Part model, mm, in its own coordinate system. Coordinates: 2 decimals unless noted, no trailing zeros. Order: outer loops, then holes, each group sorted by start corner. A loop starts at its lowest first (then second) coordinate and runs counter-clockwise, first axis right, second up.
1) Pin check, flat tips, straight feed: pin 1 Ø2 at (y, z) = (5.5, 158.5) entering from -X; pin 2 Ø1.5 at (x, y) = (-2.5, 6) entering from +Z; pin 3 Ø4 at (y, z) = (11, 253.5) entering from +X. Stop position of each tip, or through.
2) Wall check: L1, parallel to Y at x = -2.5, z = 331; L2, parallel to Z at x = -2.25, y = 5.5; L3, parallel to X at y = 6.5, z = 51. Give the ranges that are in metal, low to high.
3) Cut at A-A (z = 213). List the corners of the cut face in (x, y).
4) Cut at B-B (z = 30). List the corners of the cut face in (x, y), and give its area (3 significant figures).
Autodesk Inventor part; units mm, degrees
ref_plane "YZ Plane" through (0, 0, 0) normal (1, 0, 0) x (0, 1, 0)
ref_plane "XZ Plane" through (0, 0, 0) normal (0, 1, 0) x (-1, 0, 0)
ref_plane "XY Plane" through (0, 0, 0) normal (0, 0, 1) x (1, 0, 0)
sketch "Sketch1" plane through (0, 0, 0) normal (0, 0, 1) x (1, 0, 0)
  circle A0 centre (-2.6438, 6.9447) radius 6.8758
  line L0 (-9.4616, 7.8359) -> (-6.8245, 12.4034)
  line L1 (-6.8245, 1.4859) -> (-9.4616, 6.0534)
  line L2 (-0.0068, 0.5947) -> (-5.2808, 0.5947)
  line L3 (4.174, 6.0534) -> (1.537, 1.4859)
  line L4 (1.537, 12.4034) -> (4.174, 7.8359)
  line L5 (-5.2808, 13.2947) -> (-0.0068, 13.2947)
  point P0 (0, 0)
  point P1 (1.537, 1.4859)
  dimension "d0" = 13.7516
  dimension "d4" = 360
extrude "Extrusion1" add sketch "Sketch1" along normal blind 457.2 contours A0 L3 L2 L1 L0 L5 L4
sketch "Sketch2" plane through (0, 0, 457.2) normal (0, 0, 1) x (1, 0, 0)
  circle A0 centre (-2.6438, 6.9447) radius 2.5527
  line L0 (-5.2808, 0.5947) -> (-0.0068, 0.5947)
  line L1 (-2.6438, 6.9447) -> (-5.2808, 0.5947) construction
  line L2 (-2.6438, 6.9447) -> (-0.0068, 0.5947) construction
  point P0 (0, 0)
  dimension "d8" = 5.1054
  dimension "d9" = 6.35
extrude "Extrusion2" cut sketch "Sketch2" against normal blind 254
equation "\"d10\" = d5"
equation "\"d5\" = 254"
properties part number "12in THUNDERSHAFT STOCK"
Geometry check:
1. pin 1: stops at x = -9.51
1. pin 2: stops at z = 203.2
1. pin 3: stops at x = 3.5
2. L1: y = 0.59 to 4.4, 9.49 to 13.29
2. L2: z = 0 to 203.2
2. L3: x = -9.51 to 4.22
3. outline: (-9.46, 6.05) - (-6.82, 1.49) arc R6.88 ccw to (-5.28, 0.59) - (-0.01, 0.59) arc R6.88 ccw to (1.54, 1.49) - (4.17, 6.05) arc R6.88 ccw to (4.17, 7.84) - (1.54, 12.4) arc R6.88 ccw to (-0.01, 13.29) - (-5.28, 13.29) arc R6.88 ccw to (-6.82, 12.4) - (-9.46, 7.84) arc R6.88 ccw to start; hole circle Ø5.11 at (-2.64, 6.94)
4. outline: (-9.46, 6.05) - (-6.82, 1.49) arc R6.88 ccw to (-5.28, 0.59) - (-0.01, 0.59) arc R6.88 ccw to (1.54, 1.49) - (4.17, 6.05) arc R6.88 ccw to (4.17, 7.84) - (1.54, 12.4) arc R6.88 ccw to (-0.01, 13.29) - (-5.28, 13.29) arc R6.88 ccw to (-6.82, 12.4) - (-9.46, 7.84) arc R6.88 ccw to start
4. area: 137 mm2
